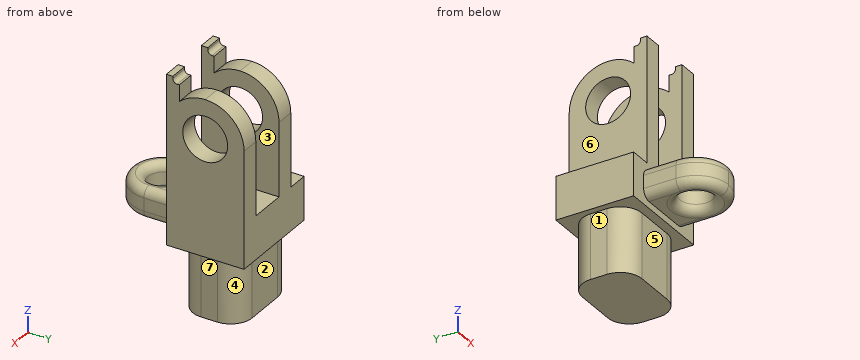
from build123d import *

# Parameters (mm, degrees)
SKETCH2_W           = 24.765
SKETCH2_H           = 17.4625
BOSS_EXTRUDE1_DEPTH = 19.05
SKETCH3_W           = 28.575
SKETCH3_H           = 22.86
BOSS_EXTRUDE2_DEPTH = 45.72
SKETCH4_W           = 6.35
SKETCH4_H           = 33.02
SKETCH4_W_2         = 11.049
CUT_EXTRUDE1_DEPTH  = 54.075706837
SKETCH5_W           = 19.05
SKETCH5_H           = 8.89
BOSS_EXTRUDE3_DEPTH = 19.05
FILLET1_R           = 9.525
SKETCH6_R           = 4.7625
CUT_EXTRUDE2_DEPTH  = 56.202869568
FILLET5_R           = 11.43
SKETCH7_R           = 6.604
CUT_EXTRUDE3_DEPTH  = 60.273091914
FILLET2_R           = 2.54
FILLET3_R           = 6.35
BOSS_EXTRUDE5_DEPTH = 5.588
BOSS_EXTRUDE6_DEPTH = 5.588
SKETCH17_W          = 1.905
SKETCH17_H          = 1.905
CUT_EXTRUDE9_DEPTH  = 63.259151384
FILLET6_R           = 1.27


# Some blends are built 0.0001 mm under size
with BuildPart() as part:
    # Sketch2 → Boss-Extrude1 (new body)
    with BuildSketch(Plane.XY):
        Rectangle(SKETCH2_W, SKETCH2_H)
    extrude(amount=-BOSS_EXTRUDE1_DEPTH)

    # Sketch3 → Boss-Extrude2 (add)
    with BuildSketch(Plane.XY):
        Rectangle(SKETCH3_W, SKETCH3_H)
    extrude(amount=BOSS_EXTRUDE2_DEPTH)

    # Sketch4 → Cut-Extrude1 (cut, through all)
    with BuildSketch(Plane(origin=(0, -11.43, 0), x_dir=(-1, 0, 0), z_dir=(0, -1, 0))):
        with Locations((11.1125, -29.21)):
            Rectangle(SKETCH4_W, SKETCH4_H)
        with Locations((-3.175, -29.21)):
            Rectangle(SKETCH4_W_2, SKETCH4_H)
    extrude(amount=-CUT_EXTRUDE1_DEPTH, mode=Mode.SUBTRACT)

    # Sketch5 → Boss-Extrude3 (add)
    with BuildSketch(Plane.XZ.offset(11.43)):
        with Locations((0, 6.4135)):
            Rectangle(SKETCH5_W, SKETCH5_H)
    extrude(amount=BOSS_EXTRUDE3_DEPTH)

    # Fillet1
    fillet1_edges = [part.edges().sort_by_distance(p)[0] for p in [
        (9.525, -30.48, 6.4135),
        (-9.525, -30.48, 6.4135),
    ]]
    fillet(fillet1_edges, radius=FILLET1_R - 0.0001)  # a hair under: the kernel refuses the full size

    # Sketch6 → Cut-Extrude2 (cut, through all)
    with BuildSketch(Plane(origin=(0, 0, 1.9685), x_dir=(-1, 0, 0), z_dir=(0, 0, -1))):
        with Locations((0, -20.955)):
            Circle(SKETCH6_R)
    extrude(amount=-CUT_EXTRUDE2_DEPTH, mode=Mode.SUBTRACT)

    # Fillet5
    fillet5_edges = [part.edges().sort_by_distance(p)[0] for p in [
        (-5.1435, -11.43, 45.72),
        (-5.1435, 11.43, 45.72),
        (11.4935, 11.43, 45.72),
        (11.4935, -11.43, 45.72),
    ]]
    fillet(fillet5_edges, radius=FILLET5_R - 0.0001)  # a hair under: the kernel refuses the full size

    # Sketch7 → Cut-Extrude3 (cut, through all)
    with BuildSketch(Plane.ZY.offset(7.9375)):
        with Locations(Location((34.29, 0, 0), (0, 0, 270))):
            Circle(SKETCH7_R)
    extrude(amount=-CUT_EXTRUDE3_DEPTH, mode=Mode.SUBTRACT)

    # Fillet2
    # the kernel refuses this fillet: 2.54 mm, written as the material it takes off along each edge
    with BuildSketch(Plane(origin=(-9.525, -11.43, 10.8585), x_dir=(0, 0, -1), z_dir=(0, -1, 0))) as fillet2_piece_1:
        with BuildLine():
            CenterArc((FILLET2_R, FILLET2_R), FILLET2_R, 180, 90)
            Line((0, FILLET2_R), (0, 0))
            Line((0, 0), (FILLET2_R, 0))
        make_face()
    extrude(amount=9.5251, mode=Mode.SUBTRACT)
    with BuildSketch(Plane(origin=(9.525, -11.43, 10.8585), x_dir=(0, 0, -1), z_dir=(0, -1, 0)), Plane(origin=(9.525, -11.43, 1.9685), x_dir=(-1, 0, 0), z_dir=(0, -1, 0)), Plane(origin=(-9.525, -11.43, 1.9685), x_dir=(0, 0, 1), z_dir=(0, -1, 0))) as fillet2_piece_2:
        with BuildLine():
            CenterArc((FILLET2_R, -FILLET2_R), FILLET2_R, 90, 90)
            Line((0, -FILLET2_R), (0, 0))
            Line((0, 0), (FILLET2_R, 0))
        make_face()
    extrude(amount=9.5251, mode=Mode.SUBTRACT)
    with BuildSketch(Plane(origin=(-0.0001, -20.9551, 10.8585), x_dir=(-1, 0, 0), z_dir=(0, 1, 0))) as fillet2_piece_3:
        with BuildLine():
            CenterArc((9.5249 - FILLET2_R, -FILLET2_R), FILLET2_R, 360, 90)
            Line((9.5249, -FILLET2_R), (9.5249, 0))
            Line((9.5249, 0), (9.5249 - FILLET2_R, 0))
        make_face()
    revolve(axis=Axis((-0.0001, -20.9551, 10.8585), (0, 0, 1)), revolution_arc=90, mode=Mode.SUBTRACT)
    with BuildSketch(Plane(origin=(0.0001, -20.9551, 10.8585), x_dir=(1, 0, 0), z_dir=(0, 1, 0))) as fillet2_piece_4:
        with BuildLine():
            CenterArc((9.5249 - FILLET2_R, FILLET2_R), FILLET2_R, 270, 90)
            Line((9.5249, FILLET2_R), (9.5249, 0))
            Line((9.5249, 0), (9.5249 - FILLET2_R, 0))
        make_face()
    revolve(axis=Axis((0.0001, -20.9551, 10.8585), (0, 0, -1)), revolution_arc=90, mode=Mode.SUBTRACT)
    with BuildSketch(Plane(origin=(-0.0001, -20.9551, 1.9685), x_dir=(-1, 0, 0), z_dir=(0, 1, 0))) as fillet2_piece_5:
        with BuildLine():
            CenterArc((9.5249 - FILLET2_R, FILLET2_R), FILLET2_R, 270, 90)
            Line((9.5249, FILLET2_R), (9.5249, 0))
            Line((9.5249, 0), (9.5249 - FILLET2_R, 0))
        make_face()
    revolve(axis=Axis((-0.0001, -20.9551, 1.9685), (0, 0, 1)), revolution_arc=90, mode=Mode.SUBTRACT)
    with BuildSketch(Plane(origin=(0.0001, -20.9551, 1.9685), x_dir=(1, 0, 0), z_dir=(0, 1, 0))) as fillet2_piece_6:
        with BuildLine():
            CenterArc((9.5249 - FILLET2_R, -FILLET2_R), FILLET2_R, 0, 90)
            Line((9.5249, -FILLET2_R), (9.5249, 0))
            Line((9.5249, 0), (9.5249 - FILLET2_R, 0))
        make_face()
    revolve(axis=Axis((0.0001, -20.9551, 1.9685), (0, 0, -1)), revolution_arc=90, mode=Mode.SUBTRACT)
    with BuildSketch(Plane(origin=(0, -20.955, 10.8585), x_dir=(-1, 0, 0), z_dir=(0, -1, 0))) as fillet2_piece_7:
        with BuildLine():
            CenterArc((4.7625 + FILLET2_R, FILLET2_R), FILLET2_R, 180, 90)
            Line((4.7625, FILLET2_R), (4.7625, 0))
            Line((4.7625, 0), (4.7625 + FILLET2_R, 0))
        make_face()
    revolve(axis=Axis((0, -20.955, 10.8585), (0, 0, -1)), mode=Mode.SUBTRACT)
    with BuildSketch(Plane(origin=(0, -20.955, 1.9685), x_dir=(-1, 0, 0), z_dir=(0, -1, 0))) as fillet2_piece_8:
        with BuildLine():
            CenterArc((4.7625 + FILLET2_R, -FILLET2_R), FILLET2_R, 90, 90)
            Line((4.7625, -FILLET2_R), (4.7625, 0))
            Line((4.7625, 0), (4.7625 + FILLET2_R, 0))
        make_face()
    revolve(axis=Axis((0, -20.955, 1.9685), (0, 0, -1)), mode=Mode.SUBTRACT)
    with BuildSketch(Plane(origin=(0.0001, -30.48, 1.9685), x_dir=(0, 1, 0), z_dir=(-1, 0, 0)), Plane(origin=(-0.0001, -30.48, 10.8585), x_dir=(0, 1, 0), z_dir=(1, 0, 0))) as fillet2_piece_9:
        with BuildLine():
            CenterArc((FILLET2_R, -FILLET2_R), FILLET2_R, 90, 90)
            Line((0, -FILLET2_R), (0, 0))
            Line((0, 0), (FILLET2_R, 0))
        make_face()
    extrude(amount=0.0002, mode=Mode.SUBTRACT)

    # Fillet3
    fillet3_edges = [part.edges().sort_by_distance(p)[0] for p in [
        (-12.3825, 8.73125, -9.525),
        (12.3825, 8.73125, -9.525),
        (12.3825, -8.73125, -9.525),
        (-12.3825, -8.73125, -9.525),
    ]]
    fillet(fillet3_edges, radius=FILLET3_R)

    # Sketch14 → Boss-Extrude5 (add)
    with BuildSketch(Plane(origin=(14.2875, 0, 0), x_dir=(0, 0, -1), z_dir=(1, 0, 0))):
        Polygon((-34.29, -11.43), (-49.53, -11.43), (-49.53, -7.62), (-42.809418994, -7.62), align=None)
    extrude(amount=-BOSS_EXTRUDE5_DEPTH)

    # Sketch16 → Boss-Extrude6 (add)
    with BuildSketch(Plane.ZY.offset(7.9375)):
        Polygon((42.809418994, -7.62), (34.29, -11.43), (49.53, -11.43), (49.53, -7.62), align=None)
    extrude(amount=-BOSS_EXTRUDE6_DEPTH)

    # Sketch17 → Cut-Extrude9 (cut, through all)
    with BuildSketch(Plane.ZY.offset(7.9375)):
        with Locations((48.5775, -8.5725)):
            Rectangle(SKETCH17_W, SKETCH17_H)
    extrude(amount=-CUT_EXTRUDE9_DEPTH, mode=Mode.SUBTRACT)

    # Fillet6
    fillet6_edges = [part.edges().sort_by_distance(p)[0] for p in [
        (-5.1435, -9.525, 47.625),
        (11.4935, -9.525, 47.625),
    ]]
    fillet(fillet6_edges, radius=FILLET6_R)


solid = part.part
Can you work these out from the model? Positions are in its coordinate system, mm. Face numbers are marked on the shaded views. A direction names the side the tool comes from. Give positions to 0.01 mm unless a question says otherwise; leave off trailing zeros. Write each loop counter-clockwise with the first axis right and the second up, starting at its lowest first coordinate (ties: lowest second). Pieces come first, ordered by that corner, then holes. Notation, with made-up numbers: M 47.5,-16.5 L 73.5,-16.5 A23 cw 73.5,5.5 Z; hole C 16.25,30.25 d3. An arc over 180 degrees is marked long. Answer in a Markdown table with one row per item. Add a question column.
Item 1: Imagine slicing it at B-B, the plane y = 4.5. Write out the boundary of the cut face in (x, z), plus the area to 3 significant figures.
Item 2: We'd pull the mould along X, two halves only. Please class the marked faces 1, 2 and 3: released by +X, released by -X, zero draft, split by the parting line, or undercut.
Item 3: Imagine slicing it at A-A, the plane z = 37.5. Write out the boundary of the cut face in (x, y), plus the area to 3 significant figures.
Item 4: On a 3-axis mill with a long thin cutter (end or side, diameter ignored), from which of +Z, -Z, +X, -X, +Y, -Y can I reach the whole of each face in a straight line? I mean the marked faces 4, 5, 6 and 7. Say none if no direction works.
Item 5: For pin 1 Ø5.5 at (x, y) = (0, -20.955) entering from +Z; pin 2 Ø9.5 at (x, z) = (-2.5, -9.5) entering from +Y; pin 3 Ø8 at (x, y) = (-9.5, 6) entering from +Z; pin 4 Ø3 at (y, z) = (-19, 4.5) entering from +X (3 decimals), each with a flat end and sliding along its axis, tell me the tip position at first contact or that it passes through.
Item 6: Please list where these lines run through material, in increasing order: L1, parallel to Z at x = -5.1, y = 0; L2, parallel to Y at x = 0, z = 6.35; L3, parallel to X at y = 7, z = 40.5.
Evaluation:
| question | item | result |
|---|---|---|
| 1 | outline | M -14.29,0 L -12.02,0 L -12.02,-19.05 L 12.02,-19.05 L 12.02,0 L 14.29,0 L 14.29,29.46 L 8.7,29.46 L 8.7,12.7 L -2.35,12.7 L -2.35,29.46 L -7.94,29.46 L -7.94,12.7 L -14.29,12.7 Z; M -7.94,39.12 L -2.35,39.12 L -2.35,44.8 L -7.94,44.8 Z; M 8.7,39.12 L 14.29,39.12 L 14.29,44.8 L 8.7,44.8 Z |
| 1 | area | 1,070 mm² |
| 2 | face 1 | released by -X |
| 2 | face 2 | zero draft |
| 2 | face 3 | undercut |
| 3 | outline | M -7.94,-11.43 L -2.35,-11.43 L -2.35,-5.77 L -7.94,-5.77 Z; M -7.94,5.77 L -2.35,5.77 L -2.35,10.97 L -7.94,10.97 Z; M 8.7,-11.43 L 14.29,-11.43 L 14.29,-5.77 L 8.7,-5.77 Z; M 8.7,5.77 L 14.29,5.77 L 14.29,10.97 L 8.7,10.97 Z |
| 3 | area | 121 mm² |
| 4 | face 4 | -Z, +X, +Y |
| 4 | face 5 | -Z, +X, -X, -Y |
| 4 | face 6 | +Z, -X, +Y, -Y |
| 4 | face 7 | -Z, +X, +Y, -Y |
| 5 | pin 1 | passes through |
| 5 | pin 2 | stops at y = 8.73 |
| 5 | pin 3 | stops at z = 45.48 |
| 5 | pin 4 | stops at x = 9.525 |
| 6 | L1 | z = -19.05 to 27.69, 40.89 to 45.72 |
| 6 | L2 | y = -30.48 to -25.72, -16.19 to 11.43 |
| 6 | L3 | x = -7.94 to -2.35, 8.7 to 14.29 |
